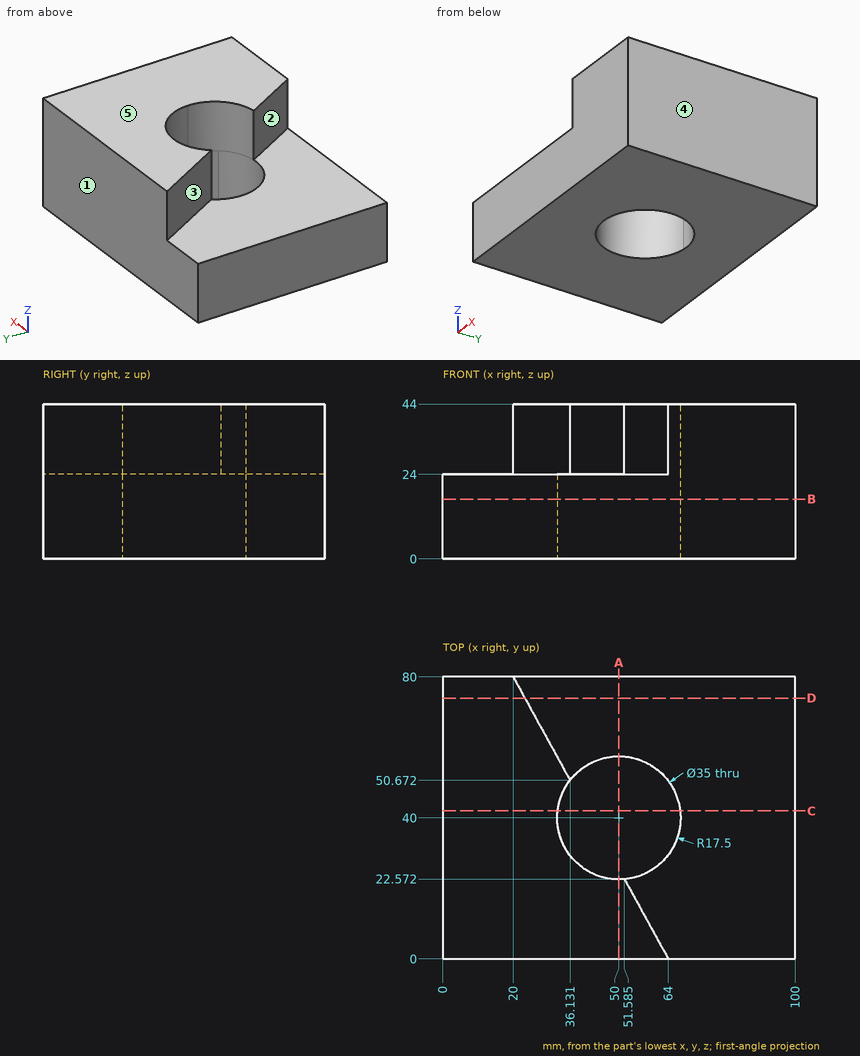
Study the drawing (mm; zero at the part's minimum x, y, z) and answer. A direction names the side the tool comes from. Give positions to 0.01 mm unless a question says otherwise; leave off trailing zeros. Loops run counter-clockwise (first coordinate to the right, second up) from the corner with the lowest first, then second, coordinate; pieces in that order, holes last. Notation, with made-up numbers: M 65.5,33 L 71.5,33 A14 cw 71.5,53 Z; hole C -7,72 d3. An arc over 180 degrees is marked long. One line per item, written item: value. Start each with the question number.
1. Find the intervals of material crossed by probe 1 along Y at (x, z) = (50, 13.25); probe 2 along X at (y, z) = (40, 15.75); probe 3 along Z at (x, y) = (5, 17), in increasing order.
2. Find section C-C (y = 42). Give the vertices of the cut face in (x, z) (1 decimal), and give its area (3 significant figures).
3. Find section A-A (x = 50). Give the vertices of the cut face in (y, z).
4. Which of the six approach directions +Z, -Z, +X, -X, +Y, -Y give full straight-line access (tool end or side, diameter ignored) to the marked faces 1 and 2?
5. Find section B-B (z = 17). Give the vertices of the cut face in (x, y) (1 decimal), and give its area (3 significant figures).
6. Each of these flat-tipped pins is pushed along its axis until it touches: P1, Ø4, axis at y = 55.5, z = 39.5, coming from the -X side (1 decimal); P2, Ø1, axis at y = 23.5, z = 21.5, coming from the -X side; P3, Ø1.5, axis at x = 50, y = 9.5, coming from the +Z side. Where does it stop, or does it pass through?
7. Determine the mould class of the marked faces 3, 4 and 5 for opening direction X: released by +X, released by -X, zero draft, split by the parting line, or undercut.
8. Find section D-D (y = 74). Give the vertices of the cut face in (x, z), and give its area (3 significant figures).
Reported:
1. probe 1: y = 0 to 22.5, 57.5 to 80
1. probe 2: x = 0 to 32.5, 67.5 to 100
1. probe 3: z = 0 to 24
2. outline: M 0,0 L 32.6,0 L 32.6,24 L 0,24 Z; M 67.4,0 L 100,0 L 100,44 L 67.4,44 Z
2. area: 2,220 mm²
3. outline: M 0,0 L 22.5,0 L 22.5,24 L 0,24 Z; M 57.5,0 L 80,0 L 80,44 L 57.5,44 Z
4. face 1: +Z, -Z, +X, -X, +Y
4. face 2: +Z, -X, -Y
5. outline: M 0,0 L 100,0 L 100,80 L 0,80 Z; hole M 63.9,29.3 A17.5 ccw 67.5,40 A17.5 ccw long Z
5. area: 7,040 mm²
6. P1: stops at x = 32.4
6. P2: stops at x = 0
6. P3: stops at z = 24
7. face 3: released by -X
7. face 4: released by +X
7. face 5: zero draft
8. outline: M 0,0 L 100,0 L 100,44 L 23.3,44 L 23.3,24 L 0,24 Z
8. area: 3,930 mm²
